```python
from build123d import *

# Parameters (mm, degrees)
F0_W     = 38.1
F0_H     = 31.75
F1_DEPTH = 38.1
F2_W     = 25.4
F2_H     = 25.4
F3_DEPTH = 12.7
F4_W     = 22.225
F4_H     = 9.525
F5_DEPTH = 38.101
F6_R     = 3.175
F7_DEPTH = 9.525
F8_R     = 0.79375


with BuildPart() as f1:
    # F0 (on Top) → F1 (new body)
    with BuildSketch(Plane.XY):
        with Locations((19.05, -15.875)):
            Rectangle(F0_W, F0_H)
    extrude(amount=F1_DEPTH)

    # F2 (on face) → F3 (cut)
    with BuildSketch(Plane.XZ.offset(31.75)):
        with Locations((25.4, 25.4)):
            Rectangle(F2_W, F2_H)
    extrude(amount=-F3_DEPTH, mode=Mode.SUBTRACT)

    # F4 (on face) → F5 (cut, through all)
    with BuildSketch(Plane.XY.offset(38.1)):
        with Locations((26.9875, -14.2875)):
            Rectangle(F4_W, F4_H)
    extrude(amount=-F5_DEPTH, mode=Mode.SUBTRACT)

    # F6 (on face) → F7 (join)
    with BuildSketch(Plane.XZ.offset(9.525)):
        with Locations((25.4, 25.4)):
            Circle(F6_R)
    extrude(amount=F7_DEPTH)

    # F8
    f8_edges = [f1.edges().sort_by_distance(p)[0] for p in [
        (22.225, -19.05, 25.4),
    ]]
    fillet(f8_edges, radius=F8_R)


solid = f1.part
```
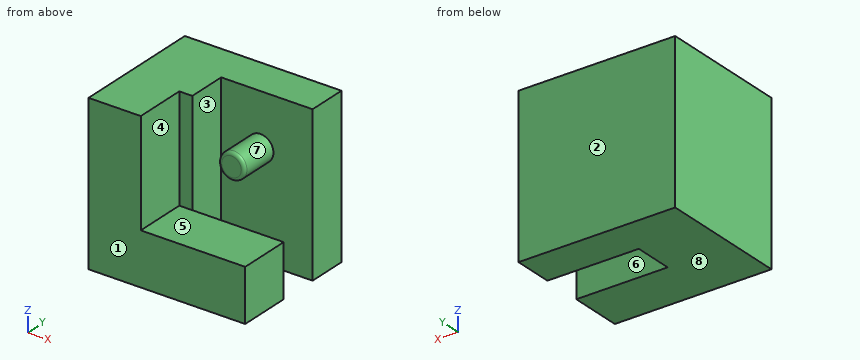
Model file for the job. Use its own axes, mm. Face numbers are marked on the shaded views. A direction names the side the tool comes from. Coordinates: 2 decimals unless noted, no trailing zeros. Write each loop counter-clockwise with the first axis right and the second up, starting at its lowest first coordinate (ties: lowest second). Pieces come first, ordered by that corner, then holes. Notation, with made-up numbers: (70.5, -7.5) - (124.5, -7.5) arc R13 ccw to (124.5, 15.5) - close; hole circle Ø10 at (-8, -13). An arc over 180 degrees is marked (long way). One line per question, with ' | ' between items. Start each with the question number.
Q1. Cut at D-D, the plane x = 32.5. List the corners of the cut face in (y, z) (3 decimals).
Q2. 3-axis set-ups, long thin cutter, end or side, ignore diameter. For the marked faces 5, 6, 7 and 8: which of +Z, -Z, +X, -X, +Y, -Y reach the whole face in a straight line?
Q3. Cut at C-C, the plane y = -29. List the corners of the cut face in (x, z), then the cut area to 3 significant figures.
Q4. Drill centre lines: line 1 (X direction, y = -13, z = 25.5) (3 decimals); line 2 (X direction, y = -16.5, z = 11) (3 decimals); line 3 (X direction, y = -21, z = 13.5). Where is each one in solid material? Low to high. Write a range as [from, to].
Q5. Pin check, flat tips, straight feed: pin 1 (3 mm diameter, centred on y = -13.5, z = 19.5, fed in from +X) (3 decimals); pin 2 (5 mm diameter, centred on x = 26.5, z = 24.5, fed in from -Y); pin 3 (4 mm diameter, centred on y = -24.5, z = 24.5, fed in from +X). Stop position of each tip, or through.
Q6. Pull direction Y, two halves, no side cores. Call the marked faces 1, 2, 3 and 4: pulls with the +Y half, pulls with the -Y half, needs draft (parallel to the pull), parting line crosses it, or undercut.
Answer below:
1) outline: (-31.75, 0) - (-19.05, 0) - (-19.05, 12.7) - (-31.75, 12.7) - close; (-9.525, 0) - (0, 0) - (0, 38.1) - (-9.525, 38.1) - close
2) face 5: +Z, +X, -Y | face 6: -Z, +X | face 7: -Y | face 8: -Z, +X, -X, +Y, -Y
3) outline: (0, 0) - (38.1, 0) - (38.1, 12.7) - (12.7, 12.7) - (12.7, 38.1) - (0, 38.1) - close | area: 806 mm^2
4) line 1: [0, 15.875], [22.227, 28.573] | line 2: [0, 15.875] | line 3: [0, 12.7]
5) pin 1: x = 15.875 | pin 2: y = -19.05 | pin 3: x = 12.7
6) face 1: pulls with the -Y half | face 2: pulls with the +Y half | face 3: undercut | face 4: needs draft
